Read the model definition and answer for the solid it produces. Units are mm, in the model's axes. A direction names the side the tool comes from. Coordinates: 2 decimals unless noted, no trailing zeros. Write each loop counter-clockwise with the first axis right and the second up, starting at its lowest first coordinate (ties: lowest second). Pieces come first, ordered by that corner, then holes.
(1) The part is cut by section C-C, the plane z = 33. Determine the outline of the cut face in (x, y).
(2) The part is cut by section D-D, the plane y = 17. Determine the outline of the cut face in (x, z).
(3) The part is cut by section B-B, the plane x = 36. Determine the outline of the cut face in (y, z), and give its area (3 significant figures).
(4) Given pin 1 (1.6 mm diameter, centred on x = 7.5, y = 6, fed in from -Z); pin 2 (1.5 mm diameter, centred on y = 10, z = -3, fed in from -X); pin 3 (6 mm diameter, centred on x = 28, z = 22, fed in from -Y), each flat-ended and moving along its own axis, determine where each tip first touches the part or whether it passes through.
(5) Determine the mould class of faces 6 (the flat face through (7, 7, 46.5)), 7 (the flat face through (3, 0, 25)), 8 (the flat face through (36, -5, 38)), 9 (the cylindrical face through (3.7, -2.465, 39.204)) for opening direction Z: pulls with the +Z half, pulls with the -Z half, needs draft (parallel to the pull), parting line crosses it, or undercut.
(6) Which of the six approach directions +Z, -Z, +X, -X, +Y, -Y give full straight-line access (tool end or side, diameter ignored) to faces 1 (the flat face through (33.5, 7, 23)), 2 (the flat face through (6.5, 7, 23)), 3 (the flat face through (8, 7, 49)), 4 (the flat face through (20, 18.4, 24)), 5 (the flat face through (20, 9, -2))?
(7) The part is cut by section A-A, the plane y = 3. Determine the outline of the cut face in (x, z), and give its area (4 significant figures).
(8) Straight lines are drawn through the part: line 1 along X through (y, z) = (14, 14.5); line 2 along Y through (x, z) = (7, 21); line 3 along X through (y, z) = (1, 47). For each, find the intervals that lie inside material, in ascending order.
```python
from build123d import *

# Parameters (mm, degrees)
SKETCH_1_W               = 40
SKETCH_1_H               = 18.4
EXTRUDE_1_DEPTH          = 46.5
CUT_EXTRUDE_1_DEPTH      = 65.037567099
CUT_EXTRUDE_1_DEPTH_BACK = 65.037567099
SKETCH_2_W               = 27
SKETCH_2_H               = 14.4
SKETCH_3_W               = 1.5
SKETCH_3_H               = 14.4
EXTRUDE_2_DEPTH          = 5
SKETCH_4_W               = 13.5
SKETCH_4_H               = 14.4
EXTRUDE_3_DEPTH          = 5
SKETCH_6_R               = 1
EXTRUDE_4_DEPTH          = 5


with BuildPart() as part:
    # 스케치1 → 보스-돌출1 (new body)
    with BuildSketch(Plane.XY):
        with Locations((20, 9.2)):
            Rectangle(SKETCH_1_W, SKETCH_1_H)
    extrude(amount=EXTRUDE_1_DEPTH)

    # 스케치2 → 컷-돌출1 (cut, two sides: drawn at the far end of the back side and taken through both)
    with BuildSketch(Plane.XY.offset(46.5).offset(-CUT_EXTRUDE_1_DEPTH_BACK)):
        with Locations((20, 7.2)):
            Rectangle(SKETCH_2_W, SKETCH_2_H)
    extrude(amount=CUT_EXTRUDE_1_DEPTH + CUT_EXTRUDE_1_DEPTH_BACK, mode=Mode.SUBTRACT)

    # 스케치3 → 보스-돌출2 (add)
    with BuildSketch(Plane.XY.offset(46.5)):
        Polygon((0, 18.4), (0, 0), (6.5, 0), (6.5, 14.4), (33.5, 14.4), (33.5, 0), (40, 0), (40, 18.4), align=None)
        with Locations((7.25, 7.2)):
            Rectangle(SKETCH_3_W, SKETCH_3_H)
        with Locations((32.75, 7.2)):
            Rectangle(SKETCH_3_W, SKETCH_3_H)
    extrude(amount=EXTRUDE_2_DEPTH)

    # 스케치4 → 보스-돌출3 (add)
    with BuildSketch(Plane(origin=(0, 0, 0), x_dir=(-1, 0, 0), z_dir=(0, 0, -1))):
        Polygon((-20, 14.4), (-20, 18.4), (-40, 18.4), (-40, 0), (-33.5, 0), (-33.5, 14.4), align=None)
        with Locations((-26.75, 7.2)):
            Rectangle(SKETCH_4_W, SKETCH_4_H)
    extrude(amount=EXTRUDE_3_DEPTH)

    # 스케치6 → 보스-돌출4 (add)
    with BuildSketch(Plane.XZ):
        with Locations(Location((36, 38.25, 0), (0, 0, 90))):
            Circle(SKETCH_6_R)
        with Locations(Location((4, 38.25, 0), (0, 0, 90))):
            Circle(SKETCH_6_R)
        with Locations(Location((4, 8.25, 0), (0, 0, 90))):
            Circle(SKETCH_6_R)
        with Locations(Location((36, 8.25, 0), (0, 0, 90))):
            Circle(SKETCH_6_R)
    extrude(amount=EXTRUDE_4_DEPTH)


solid = part.part
```
Computed:
1. outline: (0, 0) - (6.5, 0) - (6.5, 14.4) - (33.5, 14.4) - (33.5, 0) - (40, 0) - (40, 18.4) - (0, 18.4) - close
2. outline: (0, 0) - (20, 0) - (20, -5) - (40, -5) - (40, 51.5) - (0, 51.5) - close
3. outline: (-5, 7.25) - (0, 7.25) - (0, -5) - (18.4, -5) - (18.4, 51.5) - (0, 51.5) - (0, 39.25) - (-5, 39.25) - (-5, 37.25) - (0, 37.25) - (0, 9.25) - (-5, 9.25) - close
3. area: 1,060 mm2
4. pin 1: stops at z = 46.5
4. pin 2: stops at x = 20
4. pin 3: stops at y = 14.4
5. face 6: pulls with the -Z half
5. face 7: undercut
5. face 8: needs draft
5. face 9: undercut
6. face 1: -Y
6. face 2: -Z, -Y
6. face 3: +Z, -Z, -Y
6. face 4: +Z, -Z, +X, -X, +Y
6. face 5: -Z, -X, +Y, -Y
7. outline: (0, 0) - (6.5, 0) - (6.5, 46.5) - (8, 46.5) - (8, 51.5) - (0, 51.5) - close; (20, -5) - (40, -5) - (40, 51.5) - (32, 51.5) - (32, 46.5) - (33.5, 46.5) - (33.5, 0) - (20, 0) - close
7. area: 784.5 mm2
8. line 1: x = 0 to 6.5, 33.5 to 40
8. line 2: y = 14.4 to 18.4
8. line 3: x = 0 to 8, 32 to 40
